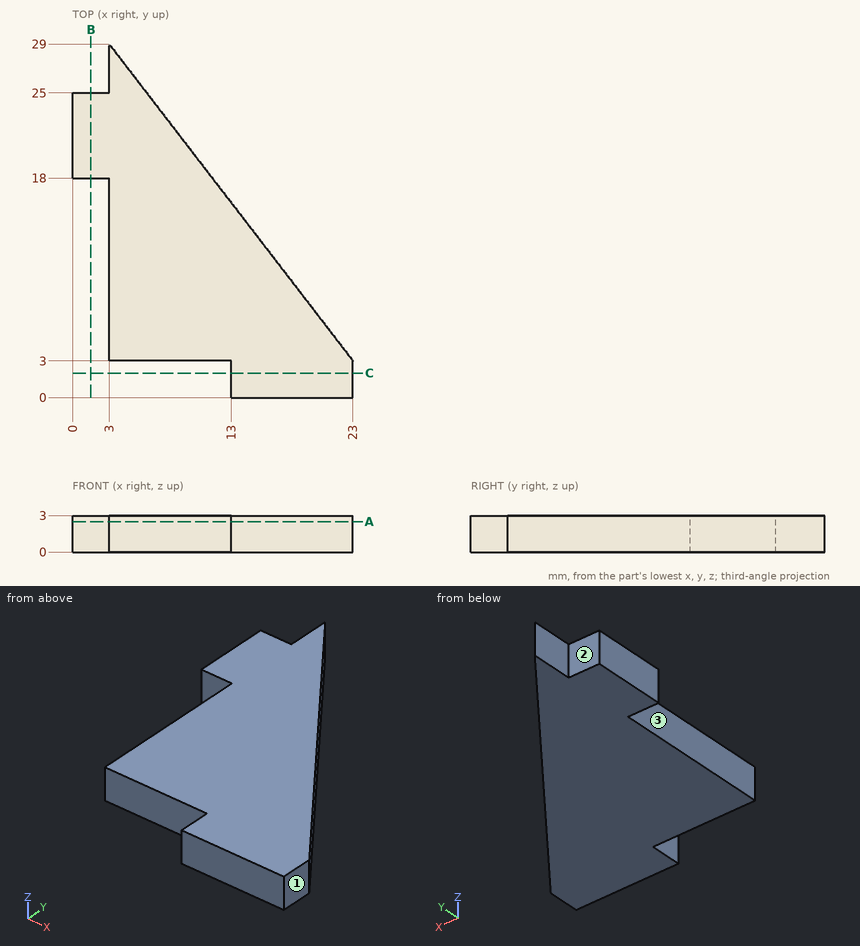
Geometry: see drawing. Coordinates: mm, zero at the bounding-box minimum. A direction names the side the tool comes from. Round coordinates to 2 decimals unless told otherwise and drop trailing zeros. Order: outer loops, then holes, each group sorted by start corner. A loop starts at its lowest first (then second) coordinate and runs counter-clockwise, first axis right, second up. Notation, with made-up numbers: (67, 85.5) - (78, 85.5) arc R35 cw to (78, 121.5) - close; hole circle Ø5 at (-3, -39). An arc over 180 degrees is marked (long way). One line per question, with ' | ' between items. Start each with the question number.
1) Set-up query: the marked faces 1, 2 and 3. Return all of +Z, -Z, +X, -X, +Y, -Y with unobstructed straight access to the full face (end or side cutting, diameter ignored); none if empty.
2) Cut plane A-A, the plane z = 2.5. Return the cut outline in (x, y).
3) Cut plane C-C, the plane y = 2. Return the cut outline in (x, z), then the cut area to 3 significant figures.
4) Contact query for flat-ended pins moving along their axis: P1, Ø1.5, axis at x = 9, z = 1.5, coming from the -Y side; P2, Ø0.9, axis at y = 12, z = 2, coming from the -X side. Output: stop coordinate, or through.
5) Cut plane B-B, the plane x = 1.5. Return the cut outline in (y, z).
6) Ray query, probe 1 along X at (y, z) = (9.5, 0.1); probe 2 along X at (y, z) = (1.75, 1.6); probe 3 along Y at (x, z) = (2.75, 1.75). Return the intervals inside material, ascending.
Worked out:
1) face 1: +Z, -Z, +X, +Y, -Y | face 2: +Z, -Z, -X, +Y | face 3: +Z, -Z, -X, -Y
2) outline: (0, 18) - (3, 18) - (3, 3) - (13, 3) - (13, 0) - (23, 0) - (23, 3) - (3, 29) - (3, 25) - (0, 25) - close
3) outline: (13, 0) - (23, 0) - (23, 3) - (13, 3) - close | area: 30.0 mm^2
4) P1: stops at y = 3 | P2: stops at x = 3
5) outline: (18, 0) - (25, 0) - (25, 3) - (18, 3) - close
6) probe 1: x = 3 to 18 | probe 2: x = 13 to 23 | probe 3: y = 18 to 25
